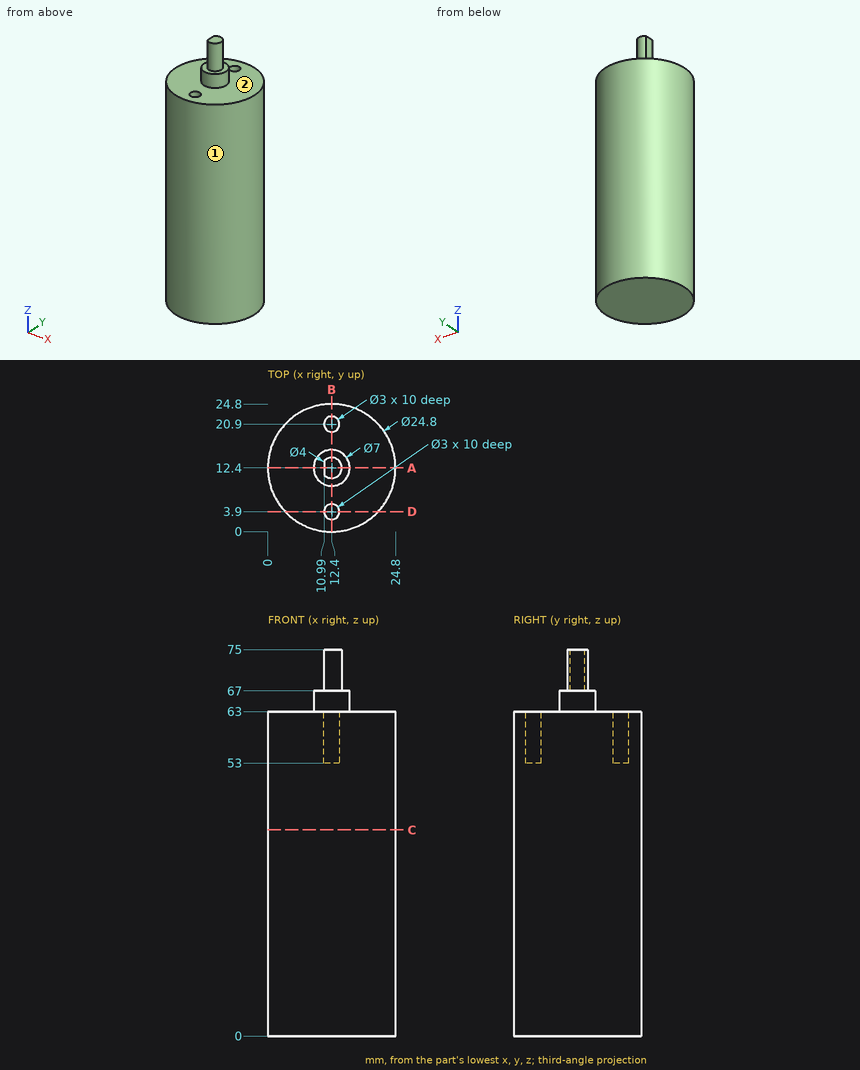
Answer from the drawing. Dimensions are ordinates in mm from the lowest x, y and z of the part. A direction names the side the tool comes from. Coordinates: 2 decimals unless noted, no trailing zeros. Loops run counter-clockwise (first coordinate to the right, second up) from the corner with the lowest first, then second, coordinate; pieces in that order, holes last. Notation, with made-up numbers: (10.5, -28.75) -> (40.5, -28.75) arc R16 ccw to (40.5, -7.75) -> close; hole circle Ø3 at (-38.5, 52.5). An arc over 180 degrees is marked (long way). Answer in a Markdown table with one row per item.
Item 1: Each of these flat-tipped pins is pushed along its axis until it touches: P1, Ø1.5, axis at y = 7.5, z = 26.5, coming from the +X side; P2, Ø8, axis at x = 5, y = 4, coming from the -Z side; P3, Ø2, axis at x = 3, z = 19, coming from the -Y side; P4, Ø4, axis at y = 8.5, z = 50.5, coming from the -X side. Where does it stop, or does it pass through?
Returned:
| item | result |
|---|---|
| P1 | stops at x = 24.08 |
| P2 | stops at z = 0 |
| P3 | stops at y = 3.28 |
| P4 | stops at x = 0.15 |
Item 2: A cutting plane is placed at D-D on y = 3.9. Determine the outline of the cut face in (x, z).
Returned:
| item | result |
|---|---|
| outline | (3.37, 0) -> (21.43, 0) -> (21.43, 63) -> (13.9, 63) -> (13.9, 53) -> (10.9, 53) -> (10.9, 63) -> (3.37, 63) -> close |
Item 3: For the marked faces 1 and 2, determine the directions among +Z, -Z, +X, -X, +Y, -Y from which every point of the face is accessible in a straight line to the end or side of a thin tool.
Returned:
| item | result |
|---|---|
| face 1 | +Z, -Z |
| face 2 | +Z |
Item 4: A cutting plane is placed at C-C on z = 40. Determine the outline of the cut face in (x, y), plus the area to 3 significant figures.
Returned:
| item | result |
|---|---|
| outline | circle Ø24.8 at (12.4, 12.4) |
| area | 483 mm^2 |
Item 5: Straight lines are drawn through the part: line 1 along Y through (x, z) = (12.4, 56.75); line 2 along Z through (x, y) = (19.5, 16); line 3 along Z through (x, y) = (14, 10.25). For each, find the intervals that lie inside material, in ascending order. Write a range as [from, to].
Returned:
| item | result |
|---|---|
| line 1 | y = [0, 2.4], [5.4, 19.4], [22.4, 24.8] |
| line 2 | z = [0, 63] |
| line 3 | z = [0, 67] |
Item 6: A cutting plane is placed at B-B on x = 12.4. Determine the outline of the cut face in (y, z).
Returned:
| item | result |
|---|---|
| outline | (0, 0) -> (24.8, 0) -> (24.8, 63) -> (22.4, 63) -> (22.4, 53) -> (19.4, 53) -> (19.4, 63) -> (15.9, 63) -> (15.9, 67) -> (14.4, 67) -> (14.4, 75) -> (10.4, 75) -> (10.4, 67) -> (8.9, 67) -> (8.9, 63) -> (5.4, 63) -> (5.4, 53) -> (2.4, 53) -> (2.4, 63) -> (0, 63) -> close |
Item 7: A cutting plane is placed at A-A on y = 12.4. Determine the outline of the cut face in (x, z).
Returned:
| item | result |
|---|---|
| outline | (0, 0) -> (24.8, 0) -> (24.8, 63) -> (15.9, 63) -> (15.9, 67) -> (14.4, 67) -> (14.4, 75) -> (10.99, 75) -> (10.99, 67) -> (8.9, 67) -> (8.9, 63) -> (0, 63) -> close |
